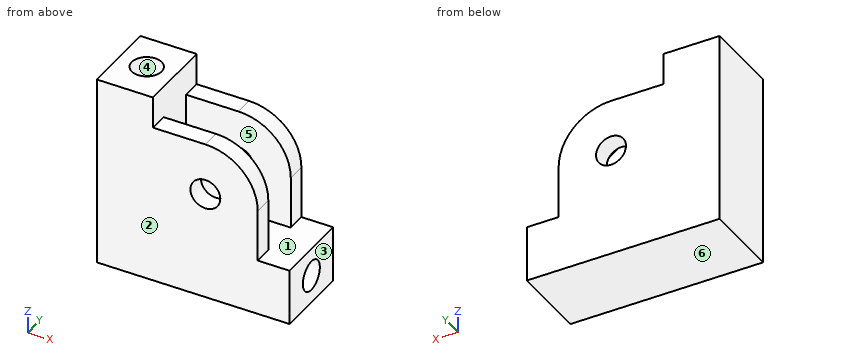
```python
from build123d import *

# Parameters (mm, degrees)
SKETCH1_W           = 8
SKETCH1_H           = 40
SKETCH1_W_2         = 40
SKETCH1_H_2         = 8
BOSS_EXTRUDE1_DEPTH = 20.6
SKETCH1_3_R         = 4
BOSS_EXTRUDE2_DEPTH = 5
BOSS_EXTRUDE4_START = 15.6
SKETCH1_4_R         = 4
BOSS_EXTRUDE4_DEPTH = 5
SKETCH2_R           = 4
CUT_EXTRUDE1_DEPTH  = 40
CHAMFER1_SIZE       = 1
SKETCH5_R           = 4
CUT_EXTRUDE7_DEPTH  = 40
CHAMFER2_SIZE       = 1


with BuildPart() as part:
    # Sketch1 → Boss-Extrude1 (new body)
    with BuildSketch(Plane(origin=(0, 0, 0), x_dir=(1, 0, 0), z_dir=(0, 1, 0))):
        Polygon((-49.993785762, 7.13734227), (-49.993785762, 47.13734227), (-41.993785762, 47.13734227), (-41.993785762, 55.13734227), (-1.993785762, 55.13734227), (-1.993785762, 58.63734227), (-53.493785762, 58.63734227), (-53.493785762, 7.13734227), align=None)
        with Locations((-45.993785762, 27.13734227)):
            Rectangle(SKETCH1_W, SKETCH1_H)
        Polygon((-1.993785762, 47.13734227), (-41.993785762, 47.13734227), (-41.993785762, 7.13734227), (-38.493785762, 7.13734227), (-38.493785762, 15.63734227), (-38.493785762, 43.63734227), (-10.493785762, 43.63734227), (-1.993785762, 43.63734227), align=None)
        with Locations((-21.993785762, 51.13734227)):
            Rectangle(SKETCH1_W_2, SKETCH1_H_2)
    extrude(amount=BOSS_EXTRUDE1_DEPTH)

    # Sketch1<3> → Boss-Extrude2 (add)
    with BuildSketch(Plane(origin=(0, 0, 0), x_dir=(1, 0, 0), z_dir=(0, 1, 0))):
        with BuildLine():
            Line((-38.493785762, 43.63734227), (-38.493785762, 15.63734227))
            Line((-38.493785762, 15.63734227), (-24.493785762, 15.63734227))
            ThreePointArc((-24.493785762, 15.63734227), (-14.594290825, 19.737847333), (-10.493785762, 29.63734227))
            Line((-10.493785762, 29.63734227), (-10.493785762, 43.63734227))
            Line((-10.493785762, 43.63734227), (-38.493785762, 43.63734227))
        make_face()
        with Locations(Location((-24.493785762, 29.63734227, 0), (0, 0, 270))):
            Circle(SKETCH1_3_R, mode=Mode.SUBTRACT)
    extrude(amount=BOSS_EXTRUDE2_DEPTH)

    # Sketch1<4> → Boss-Extrude4 (add)
    with BuildSketch(Plane(origin=(0, 0, 0), x_dir=(1, 0, 0), z_dir=(0, 1, 0)).offset(BOSS_EXTRUDE4_START)):
        with BuildLine():
            Line((-38.493785762, 43.63734227), (-38.493785762, 15.63734227))
            Line((-38.493785762, 15.63734227), (-24.493785762, 15.63734227))
            ThreePointArc((-24.493785762, 15.63734227), (-14.594290825, 19.737847333), (-10.493785762, 29.63734227))
            Line((-10.493785762, 29.63734227), (-10.493785762, 43.63734227))
            Line((-10.493785762, 43.63734227), (-38.493785762, 43.63734227))
        make_face()
        with Locations(Location((-24.493785762, 29.63734227, 0), (0, 0, 270))):
            Circle(SKETCH1_4_R, mode=Mode.SUBTRACT)
    extrude(amount=BOSS_EXTRUDE4_DEPTH)

    # Sketch2 → Cut-Extrude1 (cut)
    with BuildSketch(Plane.XY.offset(-7.13734227)):
        with Locations((-45.993785762, 10.3)):
            Circle(SKETCH2_R)
    extrude(amount=-CUT_EXTRUDE1_DEPTH, mode=Mode.SUBTRACT)

    # Chamfer1
    chamfer1_edges = [part.edges().sort_by_distance(p)[0] for p in [
        (-49.993785762, 10.3, -47.13734227),
    ]]
    chamfer(chamfer1_edges, length=CHAMFER1_SIZE)

    # Sketch5 → Cut-Extrude7 (cut)
    with BuildSketch(Plane(origin=(-1.993785762, 0, 0), x_dir=(0, 0, -1), z_dir=(1, 0, 0))):
        with Locations((51.13734227, 10.3)):
            Circle(SKETCH5_R)
    extrude(amount=-CUT_EXTRUDE7_DEPTH, mode=Mode.SUBTRACT)

    # Chamfer2
    chamfer2_edges = [part.edges().sort_by_distance(p)[0] for p in [
        (-41.993785762, 10.3, -47.13734227),
    ]]
    chamfer(chamfer2_edges, length=CHAMFER2_SIZE)


solid = part.part
```
Geometry check sheet. Reference: the model listing, model coordinates, mm. Face numbers are marked on the shaded views. A direction names the side the tool comes from. Coordinates: 2 decimals unless noted, no trailing zeros. Loops run counter-clockwise (first coordinate to the right, second up) from the corner with the lowest first, then second, coordinate; pieces in that order, holes last. Notation, with made-up numbers: (-5.5, -39) - (46.5, -39) arc R17 ccw to (46.5, -7) - close; hole circle Ø10 at (-11.75, 20). An arc over 180 degrees is marked (long way). One line per item, written item: value. Start each with the question number.
(1) Cross-section at A-A on z = -36. Enter the section's corners in (x, y), plus the area to 3 significant figures.
(2) Mould release check, pull along Y, two halves, no side actions. Record for the marked faces 1, 2 and 3: released by +Y, released by -Y, zero draft, split by the parting line, or undercut.
(3) Material ranges on line 1 (Z direction, x = -21.5, y = 10); line 2 (Y direction, x = -20, z = -20); line 3 (X direction, y = 1.75, z = -15.5), recorded low to high. Write a range as [from, to].
(4) Cross-section at C-C on y = 3.75. Enter the section's corners in (x, z).
(5) Depth check by flat-ended pin: P1, Ø10.5, axis at x = -24.49, z = -29.64, coming from the +Y side; P2, Ø3, axis at y = 10.5, z = -15.5, coming from the +X side; P3, Ø4, axis at y = 3.5, z = -37.5, coming from the +X side; P4, Ø6.5, axis at x = -24.49, z = -29.64, coming from the -Y side. Enter the tip coordinate at first touch or a pass-through.
(6) Cross-section at D-D on y = 10.3. Enter the section's corners in (x, z), plus the area to 3 significant figures.
(7) Cross-section at B-B on x = -30. Enter the section's corners in (y, z), plus the area to 3 significant figures.
(8) Tool access check on the marked faces 4, 5 and 6. Record the directions out of +Z, -Z, +X, -X, +Y, -Y that give a thin tool (end or side, any length) a straight path to the whole face; none if there is none.
Results below:
1. outline: (-53.49, 0) - (-10.49, 0) - (-10.49, 5) - (-38.49, 5) - (-38.49, 15.6) - (-10.49, 15.6) - (-10.49, 20.6) - (-53.49, 20.6) - close; hole circle Ø8 at (-45.99, 10.3)
1. area: 539 mm2
2. face 1: undercut
2. face 2: released by -Y
2. face 3: zero draft
3. line 1: z = [-58.64, -55.13], [-47.15, -43.64]
3. line 2: y = [0, 5], [15.6, 20.6]
3. line 3: x = [-53.49, -38.49]
4. outline: (-53.49, -58.64) - (-1.99, -58.64) - (-1.99, -43.64) - (-10.49, -43.64) - (-10.49, -29.64) arc R14 ccw to (-24.49, -15.64) - (-38.49, -15.64) - (-38.49, -7.14) - (-53.49, -7.14) - close; hole circle Ø8 at (-24.49, -29.64)
5. P1: stops at y = 20.6
5. P2: stops at x = -38.49
5. P3: stops at x = -10.49
5. P4: passes through
6. outline: (-53.49, -58.64) - (-1.99, -58.64) - (-1.99, -55.14) - (-40.99, -55.14) - (-41.99, -54.14) - (-41.99, -48.14) - (-40.99, -47.14) - (-1.99, -47.14) - (-1.99, -43.64) - (-38.49, -43.64) - (-38.49, -7.14) - (-41.99, -7.14) - (-41.99, -46.14) - (-42.99, -47.14) - (-48.99, -47.14) - (-49.99, -46.14) - (-49.99, -7.14) - (-53.49, -7.14) - close
6. area: 682 mm2
7. outline: (0, -58.64) - (20.6, -58.64) - (20.6, -15.64) - (15.6, -15.64) - (15.6, -43.64) - (5, -43.64) - (5, -15.64) - (0, -15.64) - close; hole circle Ø8 at (10.3, -51.14)
7. area: 539 mm2
8. face 4: +Z
8. face 5: +Z, +X
8. face 6: -Z, +X, -X, +Y, -Y
